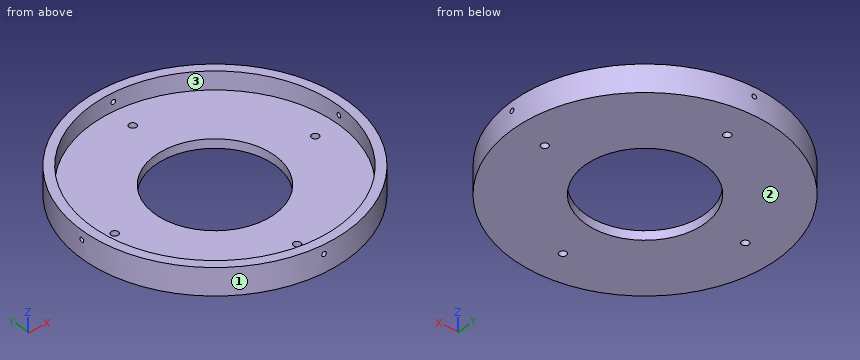
from build123d import *

# Parameters (mm, degrees)
SKETCH1_R               = 73
SKETCH1_R_2             = 33
BOSS_EXTRUDE1_DEPTH     = 5
SKETCH2_R               = 73
SKETCH2_R_2             = 68
BOSS_EXTRUDE2_DEPTH     = 10
CUT_EXTRUDE1_REACH      = 106.322
CUT_EXTRUDE1_END_RADIUS = 73
SKETCH3_R               = 1.25
CIRPATTERN1_COUNT       = 4
F_4_0MM_DOWEL_HOLE1_D   = 4


with BuildPart() as part:
    # Sketch1 → Boss-Extrude1 (new body)
    with BuildSketch(Plane.XY):
        Circle(SKETCH1_R)
        Circle(SKETCH1_R_2, mode=Mode.SUBTRACT)
    extrude(amount=BOSS_EXTRUDE1_DEPTH)

    # Sketch2 → Boss-Extrude2 (add)
    with BuildSketch(Plane.XY.offset(5)):
        Circle(SKETCH2_R)
        Circle(SKETCH2_R_2, mode=Mode.SUBTRACT)
    extrude(amount=BOSS_EXTRUDE2_DEPTH)

    # Cut-Extrude1: up to this cylinder (the profile starts inside it)
    cut_extrude1_end = Plane(origin=(0, 0, 10), z_dir=(0, 0, -1)) * Cylinder(CUT_EXTRUDE1_END_RADIUS, 359.644, mode=Mode.PRIVATE)
    # Sketch3 → Cut-Extrude1 (cut, up to the surface)
    with BuildSketch(Plane(origin=(0, 0, 0), x_dir=(1, 0, 0), z_dir=(0, 1, 0)), mode=Mode.PRIVATE) as cut_extrude1_sk1:
        with Locations(Location((0, -10, 0), (0, 0, 270))):
            Circle(SKETCH3_R)
    cut_extrude1_tool1 = extrude(cut_extrude1_sk1.sketch, amount=-CUT_EXTRUDE1_REACH, mode=Mode.PRIVATE) & cut_extrude1_end
    cut_extrude1 = cut_extrude1_tool1.solids().sort_by_distance((0, 0, 10))[0]
    add(cut_extrude1, mode=Mode.SUBTRACT)

    # CirPattern1: Cut-Extrude1 ×4 about axis
    cirpattern1_axis = Axis((0, 0, 5), (0, 0, -1))
    for i in range(1, CIRPATTERN1_COUNT):
        add(cut_extrude1.rotate(cirpattern1_axis, i * 360 / CIRPATTERN1_COUNT), mode=Mode.SUBTRACT)

    # Ø4.0mm Dowel Hole1 (through all)
    with Locations(Plane(origin=(0, 0, 0), x_dir=(-1, 0, 0), z_dir=(0, 0, -1))):
        with Locations((0, 55), (55, 0), (0, -55), (-55, 0)):
            Hole(F_4_0MM_DOWEL_HOLE1_D / 2)


solid = part.part
For this review, take the finished solid that the model builds, in its own axes (mm). Face numbers are marked on the shaded views. Give positions to 0.01 mm unless a question says otherwise; leave off trailing zeros. Order: outer loops, then holes, each group sorted by start corner. A loop starts at its lowest first (then second) coordinate and runs counter-clockwise, first axis right, second up. Notation, with made-up numbers: (57, -3.75) - (104, -3.75) arc R9 ccw to (104, 9.25) - close; hole circle Ø10 at (22, 59). An arc over 180 degrees is marked (long way). Answer as a JSON object with one key per item and string values. Group by question number.
Item 1: Clearance check with flat-ended pins moving along their axes: pin 1 Ø4.5 at (x, y) = (55, 0) entering from +Z; pin 2 Ø2.5 at (x, y) = (0, -55) entering from +Z; pin 3 Ø1.5 at (x, z) = (36, 3) entering from -Y; pin 4 Ø2 at (y, z) = (-45, 11.5) entering from -X. State where each tip first meets the part, or that it passes through.
Item 2: Take a section at D-D on y = -50. Give the boundary of the cut face in (x, z).
Item 3: Draft analysis for pull direction X (two halves, no side actions). For the marked faces 1, 2 and 3, state which applies: pulls with the +X half, pulls with the -X half, needs draft (parallel to the pull), parting line crosses it, or undercut.
Item 4: Wall thickness on line 1 along Y through (x, z) = (0, 2.7); line 2 along Y through (x, z) = (1.5, 2.25); line 3 along Z through (x, y) = (0, 70): over which ranges is each line inside the solid? List them lowest first.
Item 5: Take a section at C-C on z = 1.75. Give the boundary of the cut face in (x, y), and give its area (3 significant figures).
Item 6: Take a section at B-B on y = 17.5. Give the boundary of the cut face in (x, z).
Item 7: Take a section at A-A on x = 27.5. Give the boundary of the cut face in (y, z), and give its area (3 significant figures).
Reported:
{
 "1": {"pin 1": "z = 5", "pin 2": "through", "pin 3": "y = -63.93", "pin 4": "x = -58.25"},
 "2": {"outline": "(-53.19, 0) - (53.19, 0) - (53.19, 15) - (46.09, 15) - (46.09, 5) - (-46.09, 5) - (-46.09, 15) - (-53.19, 15) - close"},
 "3": {"face 1": "parting line crosses it", "face 2": "needs draft", "face 3": "undercut"},
 "4": {"line 1": "-73 to -57, -53 to -33, 33 to 53, 57 to 73", "line 2": "-72.98 to -56.32, -53.68 to -32.97, 32.97 to 53.68, 56.32 to 72.98", "line 3": "0 to 8.75, 11.25 to 15"},
 "5": {"outline": "circle Ø146 at (0, 0); hole circle Ø4 at (-55, 0); hole circle Ø66 at (0, 0); hole circle Ø4 at (0, -55); hole circle Ø4 at (0, 55); hole circle Ø4 at (55, 0)", "area": "13,300 mm^2"},
 "6": {"outline": "(-70.87, 0) - (-27.98, 0) - (-27.98, 5) - (-65.71, 5) - (-65.71, 15) - (-70.87, 15) - close; (27.98, 0) - (70.87, 0) - (70.87, 15) - (65.71, 15) - (65.71, 5) - (27.98, 5) - close"},
 "7": {"outline": "(-67.62, 0) - (-18.24, 0) - (-18.24, 5) - (-62.19, 5) - (-62.19, 15) - (-67.62, 15) - close; (18.24, 0) - (67.62, 0) - (67.62, 15) - (62.19, 15) - (62.19, 5) - (18.24, 5) - close", "area": "602 mm^2"}
}
